Print and shaded views of the part. All mm, measured from the part's lowest x, y and z. Round coordinates to 2 decimals unless told otherwise and drop trailing zeros. Write each loop counter-clockwise with the first axis right and the second up, starting at its lowest first coordinate (ties: lowest second). Pieces come first, ordered by that corner, then holes. Notation, with made-up numbers: (35, 71) - (71, 71) arc R29 ccw to (71, 109) - close; hole circle Ø10 at (4.25, 6.5). An arc over 180 degrees is marked (long way). Answer as a JSON object with one key per item and string values. Group by question number.
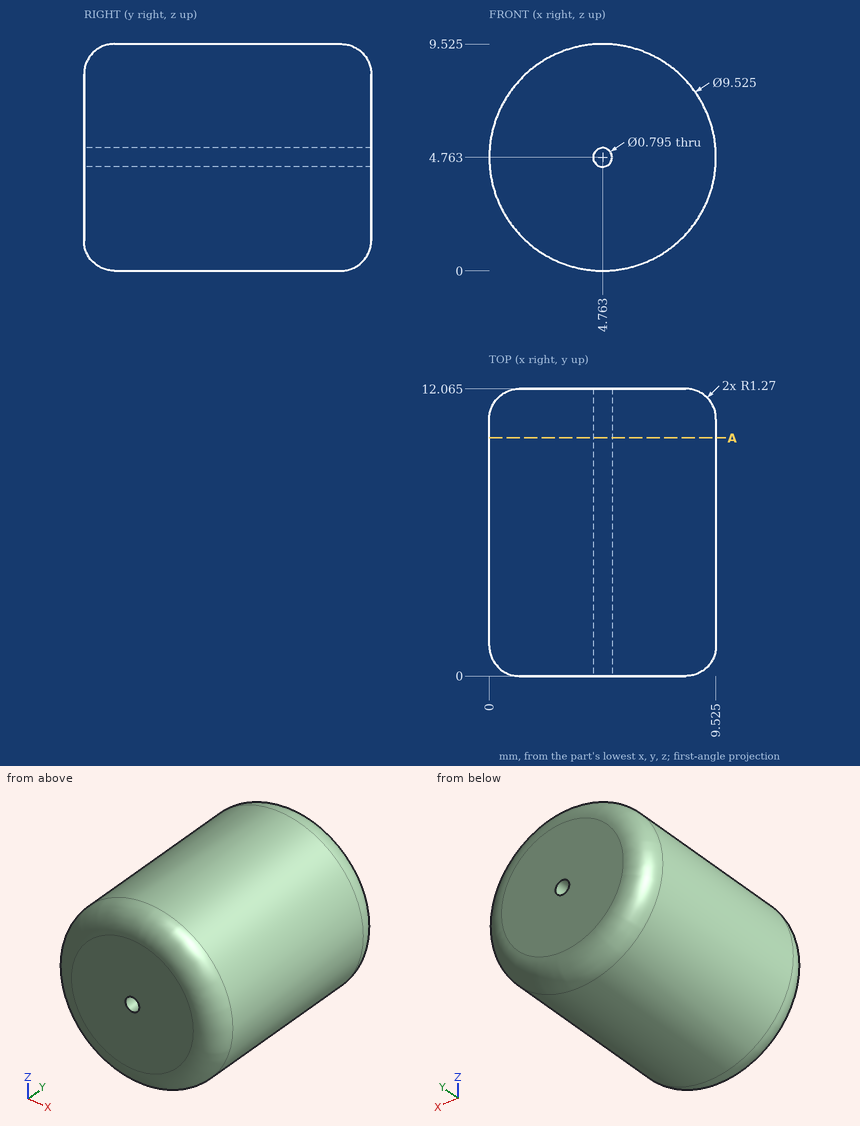
(1) Slice it at A-A (y = 10). Write the cut outline in (x, z) (1 decimal).
(2) Drill centre lines: line 1 (X direction, y = 7, z = 4.5) (1 decimal); line 2 (Z direction, x = 5, y = 4.25) (1 decimal); line 3 (Y direction, x = 1.25, z = 5.5). Where is each one in solid material? Low to high. Write a range as from..to.
(3) Flat gauge pins, fed straight in: pin 1 (4 mm diameter, centred on y = 6.5, z = 8, fed in from -X); pin 2 (1.5 mm diameter, centred on x = 2.5, y = 7, fed in from +Z); pin 3 (1.5 mm diameter, centred on y = 4, z = 8, fed in from +X) (1 decimal). Where does each tip first touch, or does it go through?
Answer:
{
 "1": {"outline": "circle Ø9.5 at (4.8, 4.8); hole circle Ø0.8 at (4.8, 4.8)"},
 "2": {"line 1": "0..4.5, 5.1..9.5", "line 2": "0..4.4, 5.1..9.5", "line 3": "0..12.06"},
 "3": {"pin 1": "x = 0.16", "pin 2": "z = 9.28", "pin 3": "x = 8.8"}
}
